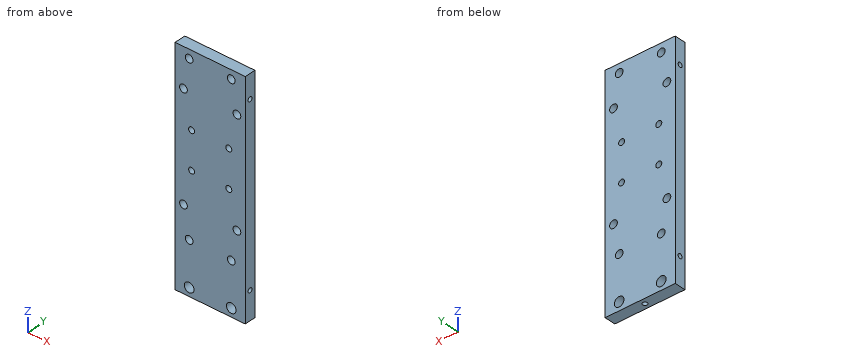
```python
from build123d import *

# Parameters (mm, degrees)
SKETCH1_W               = 40
SKETCH1_H               = 160
BOSS_EXTRUDE1_DEPTH     = 3.175
M4_5_THROUGH_DEPTH      = 6.35
M4_5_THROUGH_DEPTH_BACK = 3.175
SKETCH3_R               = 2.75
SKETCH3_R_2             = 2.2
SKETCH4_R               = 1.3
M3_DRILL_DEPTH          = 8
SKETCH5_R               = 2.2
M4_THROUGH_DEPTH        = 6.35
M4_DRILL_DEPTH          = 3.175
M4_DRILL_DEPTH_BACK     = 10
SKETCH6_R               = 1.7
SKETCH7_W               = 40
SKETCH7_H               = 30.2375
CUT_EXTRUDE2_DEPTH      = 6.35
SKETCH8_R               = 1.3
CUT_EXTRUDE3_DEPTH      = 8


with BuildPart() as part:
    # Sketch1 → Boss-Extrude1 (new, symmetric)
    with BuildSketch(Plane(origin=(0, 0, 0), x_dir=(1, 0, 0), z_dir=(0, 1, 0))):
        Rectangle(SKETCH1_W, SKETCH1_H)
    extrude(amount=BOSS_EXTRUDE1_DEPTH, both=True)

    # Sketch3 → M4/5_through (cut, two sides: drawn at the far end of the back side and taken through both)
    with BuildSketch(Plane(origin=(0, 0, 0), x_dir=(1, 0, 0), z_dir=(0, 1, 0)).offset(-M4_5_THROUGH_DEPTH_BACK)):
        with Locations(Location((12, 75.2375, 0), (0, 0, 270))):
            Circle(SKETCH3_R)
        with Locations(Location((12, 50.2375, 0), (0, 0, 270))):
            Circle(SKETCH3_R_2)
        with Locations(Location((-12, 50.2375, 0), (0, 0, 270))):
            Circle(SKETCH3_R_2)
        with Locations(Location((-12, 75.2375, 0), (0, 0, 270))):
            Circle(SKETCH3_R)
        with Locations(Location((-12, -44.7625, 0), (0, 0, 270))):
            Circle(SKETCH3_R_2)
        with Locations(Location((12, -44.7625, 0), (0, 0, 270))):
            Circle(SKETCH3_R_2)
    extrude(amount=M4_5_THROUGH_DEPTH + M4_5_THROUGH_DEPTH_BACK, mode=Mode.SUBTRACT)

    # Sketch4 → M3_DRILL (cut)
    with BuildSketch(Plane(origin=(0, 0, -80), x_dir=(-1, 0, 0), z_dir=(0, 0, -1))):
        Circle(SKETCH4_R)
    extrude(amount=-M3_DRILL_DEPTH, mode=Mode.SUBTRACT)

    # Sketch5 → M4_through (cut)
    with BuildSketch(Plane(origin=(0, 3.175, 0), x_dir=(1, 0, 0), z_dir=(0, 1, 0))):
        with Locations(Location((-15.2375, -27.6625, 0), (0, 0, 270))):
            Circle(SKETCH5_R)
        with Locations(Location((15.2375, -27.6625, 0), (0, 0, 270))):
            Circle(SKETCH5_R)
        with Locations(Location((15.2375, 33.1375, 0), (0, 0, 270))):
            Circle(SKETCH5_R)
        with Locations(Location((-15.2375, 33.1375, 0), (0, 0, 270))):
            Circle(SKETCH5_R)
    extrude(amount=-M4_THROUGH_DEPTH, mode=Mode.SUBTRACT)

    # Sketch6 → M4_Drill (cut, two sides: drawn at the far end of the back side and taken through both)
    with BuildSketch(Plane(origin=(0, 0, 0), x_dir=(1, 0, 0), z_dir=(0, 1, 0)).offset(-M4_DRILL_DEPTH_BACK)):
        with Locations(Location((-10.606601718, 13.344101718, 0), (0, 0, 270))):
            Circle(SKETCH6_R)
        with Locations(Location((10.606601718, 13.344101718, 0), (0, 0, 270))):
            Circle(SKETCH6_R)
        with Locations(Location((10.606601718, -7.869101718, 0), (0, 0, 270))):
            Circle(SKETCH6_R)
        with Locations(Location((-10.606601718, -7.869101718, 0), (0, 0, 270))):
            Circle(SKETCH6_R)
    extrude(amount=M4_DRILL_DEPTH + M4_DRILL_DEPTH_BACK, mode=Mode.SUBTRACT)

    # Sketch7 → Cut-Extrude2 (cut)
    with BuildSketch(Plane(origin=(0, 3.175, 0), x_dir=(1, 0, 0), z_dir=(0, 1, 0))):
        with Locations((0, -64.88125)):
            Rectangle(SKETCH7_W, SKETCH7_H)
    extrude(amount=-CUT_EXTRUDE2_DEPTH, mode=Mode.SUBTRACT)

    # Sketch8 → Cut-Extrude3 (cut)
    with BuildSketch(Plane.ZY.offset(20)):
        with Locations((36.2625, 0)):
            Circle(SKETCH8_R)
        with Locations((-64, 0)):
            Circle(SKETCH8_R)
    cut_extrude3 = extrude(amount=-CUT_EXTRUDE3_DEPTH, mode=Mode.SUBTRACT)

    # Mirror1: Cut-Extrude3 across plane
    add(cut_extrude3.mirror(Plane(origin=(0, 0, 0), x_dir=(0, 0, 1), z_dir=(1, 0, 0))), mode=Mode.SUBTRACT)


solid = part.part
```
Geometry check sheet. Reference: the model listing, model coordinates, mm. Coordinates: 2 decimals unless noted, no trailing zeros. Order: outer loops, then holes, each group sorted by start corner. A loop starts at its lowest first (then second) coordinate and runs counter-clockwise, first axis right, second up. Notation, with made-up numbers: (40, 12) - (75, 12) arc R19 cw to (75, 22) - close; hole circle Ø4 at (16.5, 56). An arc over 180 degrees is marked (long way). Answer as a JSON object with one key per item and string values. Group by question number.
Item 1: Scan lines: probe 1 along Z at (x, y) = (-17.5, -0.25); probe 2 along Z at (x, y) = (-15, 2.25); probe 3 along X at (y, z) = (2.5, -34.5). Record each from-to range of solid material in increasing order.
Item 2: Sectioned sample at B-B, the plane x = 0. Record the cut outline in (y, z) (1 decimal).
Item 3: Sectioned sample at C-C, the plane y = 0. Give the number of separate pieces and of enclosed holes in the cut face, and give its area (3 significant figures).
Item 4: Depth check by flat-ended pin: pin 1 Ø1.6 at (y, z) = (0, 36.26) entering from +X; pin 2 Ø2.5 at (x, z) = (15.24, -33.14) entering from -Y; pin 3 Ø0.8 at (y, z) = (0.5, 36) entering from -X. Enter the tip coordinate at first touch or a pass-through.
Item 5: Sectioned sample at A-A, the plane z = -64. Record the cut outline in (x, y) (3 decimals).
Resolved:
{
 "1": {"probe 1": "-80 to -65.28, -62.72 to 34.99, 37.54 to 49.76", "probe 2": "-80 to -35.32, -30.95 to 25.48, 29.85 to 49.76", "probe 3": "-20 to -16.96, -13.51 to 13.51, 16.96 to 20"},
 "2": {"outline": "(-3.2, -80) - (-1.3, -80) - (-1.3, -72) - (1.3, -72) - (1.3, -80) - (3.2, -80) - (3.2, 49.8) - (-3.2, 49.8) - close"},
 "3": {"separate pieces": "1", "enclosed holes": "14", "area": "4,880 mm^2"},
 "4": {"pin 1": "x = 12", "pin 2": "through", "pin 3": "x = -12"},
 "5": {"outline": "(-20, -3.175) - (20, -3.175) - (20, -1.3) - (12, -1.3) - (12, 1.3) - (20, 1.3) - (20, 3.175) - (-20, 3.175) - (-20, 1.3) - (-12, 1.3) - (-12, -1.3) - (-20, -1.3) - close"}
}
